Autodesk Inventor part; units mm, degrees
ref_plane "YZ Plane" through (0, 0, 0) normal (1, 0, 0) x (0, 1, 0)
ref_plane "XZ Plane" through (0, 0, 0) normal (0, 1, 0) x (-1, 0, 0)
ref_plane "XY Plane" through (0, 0, 0) normal (0, 0, 1) x (1, 0, 0)
sketch "Esquisse1" plane through (0, 0, 0) normal (0, 0, 1) x (1, 0, 0)
  line L0 (-198.5, -153) -> (198.5, -153)
  line L1 (198.5, -153) -> (198.5, 153)
  line L2 (198.5, 153) -> (-198.5, 153)
  line L3 (-198.5, 153) -> (-198.5, -153)
  line L4 (-198.5, -153) -> (198.5, 153) construction
  line L5 (198.5, -153) -> (-198.5, 153) construction
  point P0 (0, 0)
  dimension "Largueur_plaque_support" = 397
  dimension "Profondeur_plaque_support" = 306
extrude "Embase" add sketch "Esquisse1" along normal mid plane 5
sketch "Trous moteur" plane through (0, 0, 2.5) normal (0, 0, 1) x (1, 0, 0)
  line L0 (-12.4135, -12.4135) -> (37.5865, 37.5865) construction
  line L1 (-12.4135, 37.5865) -> (37.5865, -12.4135) construction
  point P0 (0, 0)
  point P1 (12.5865, 12.5865)
  dimension "Entraxe_vis_moteur" = 50
  dimension "d5" = 50
  dimension "Entraxe_engrenage" = 17.8
hole "Passage vis moteur" at (-12.4135, 37.5865, 2.5) at (37.5865, 37.5865, 2.5) at (37.5865, -12.4135, 2.5) at (-12.4135, -12.4135, 2.5) direction (0, 0, -1) diameter 4.5 end through all
hole "Passage axe moteur" at (12.5865, 12.5865, 2.5) direction (0, 0, -1) diameter 21 end through all
sketch "Esquisse3" plane through (0, 0, 2.5) normal (0, 0, 1) x (1, 0, 0)
  point P0 (0, 0)
  point P1 (-16.5, 73.3)
  point P2 (-1.5, 73.3)
  dimension "Entraxe_fication" = 15
  dimension "Demi_entraxe" = 73.3
  dimension "Décalage" = 1.5
hole "Passage vis bras" at (-16.5, 73.3, 2.5) at (-1.5, 73.3, 2.5) direction (0, 0, -1) diameter 5.5 end through all
mirror "Symétrie passage vis bras" about plane through (0, 0, 0) normal (0, 1, 0) of "Passage vis bras"
sketch "Esquisse4" plane through (0, 0, 2.5) normal (0, 0, 1) x (1, 0, 0)
  point P0 (0, 0)
  point P1 (-170, 125)
  dimension "d31" = 170
  dimension "d32" = 125
hole "Perçage4" at (-170, 125, 2.5) direction (0, 0, -1) diameter 15 end through all
equation "\"d5\" = Entraxe_vis_moteur"
properties part number "Plaque support" material "Plastique PMMA"
CAD build for the part. Positions are in the model's coordinates, mm. Round coordinates to 2 decimals unless told otherwise and drop trailing zeros. Order: outer loops, then holes, each group sorted by start corner. A loop starts at its lowest first (then second) coordinate and runs counter-clockwise, first axis right, second up. Notation, with made-up numbers: (71, 84) - (115, 84) arc R34 ccw to (115, 114) - close; hole circle Ø5 at (8.25, -5.5). An arc over 180 degrees is marked (long way). Return JSON: item names as keys, results as strings.
(1) Wall check: probe 1 along Y at (x, z) = (-16.5, -0.75); probe 2 along Y at (x, z) = (14, -0.4); probe 3 along X at (y, z) = (75, 2.1). Give the ranges that are in metal, low to high. Write a range as from..to.
Answer key:
{"probe 1": "y = -153..-76.05, -70.55..70.55, 76.05..153", "probe 2": "y = -153..2.18, 22.99..153", "probe 3": "x = -198.5..-18.66, -14.34..-3.66, 0.66..198.5"}
(2) Cut at A-A (x = -170). Give the cut face in (y, z), then the cut area to 4 significant figures.
Answer key:
{"outline": "(-153, -2.5) - (117.5, -2.5) - (117.5, 2.5) - (-153, 2.5) - close; (132.5, -2.5) - (153, -2.5) - (153, 2.5) - (132.5, 2.5) - close", "area": "1,455 mm^2"}
(3) Cut at B-B (y = 125). Give the cut face in (x, z).
Answer key:
{"outline": "(-198.5, -2.5) - (-177.5, -2.5) - (-177.5, 2.5) - (-198.5, 2.5) - close; (-162.5, -2.5) - (198.5, -2.5) - (198.5, 2.5) - (-162.5, 2.5) - close"}
(4) Pull direction X, two halves, no side cores. Call faces 1 (the face through (-3, 2, -2.5)), 2 (the face through (-176.324, 120.968, -0.035)): +X half, -X half, draft (parallel to the pull), parting line (faces both ways), or undercut.
Answer key:
{"face 1": "draft", "face 2": "undercut"}
